The figure shows three views and two pictorial views of one solid part (mm, origin at its lowest corner). Answer the questions. A direction names the side the tool comes from. Coordinates: 2 decimals unless noted, no trailing zeros. Loops run counter-clockwise (first coordinate to the right, second up) from the corner with the lowest first, then second, coordinate; pieces in that order, holes last. Notation, with made-up numbers: (0.25, 33.5) - (38.25, 33.5) arc R17 ccw to (38.25, 63.5) - close; hole circle Ø7 at (34, -2). An arc over 180 degrees is marked (long way). One line per question, with ' | ' between items.
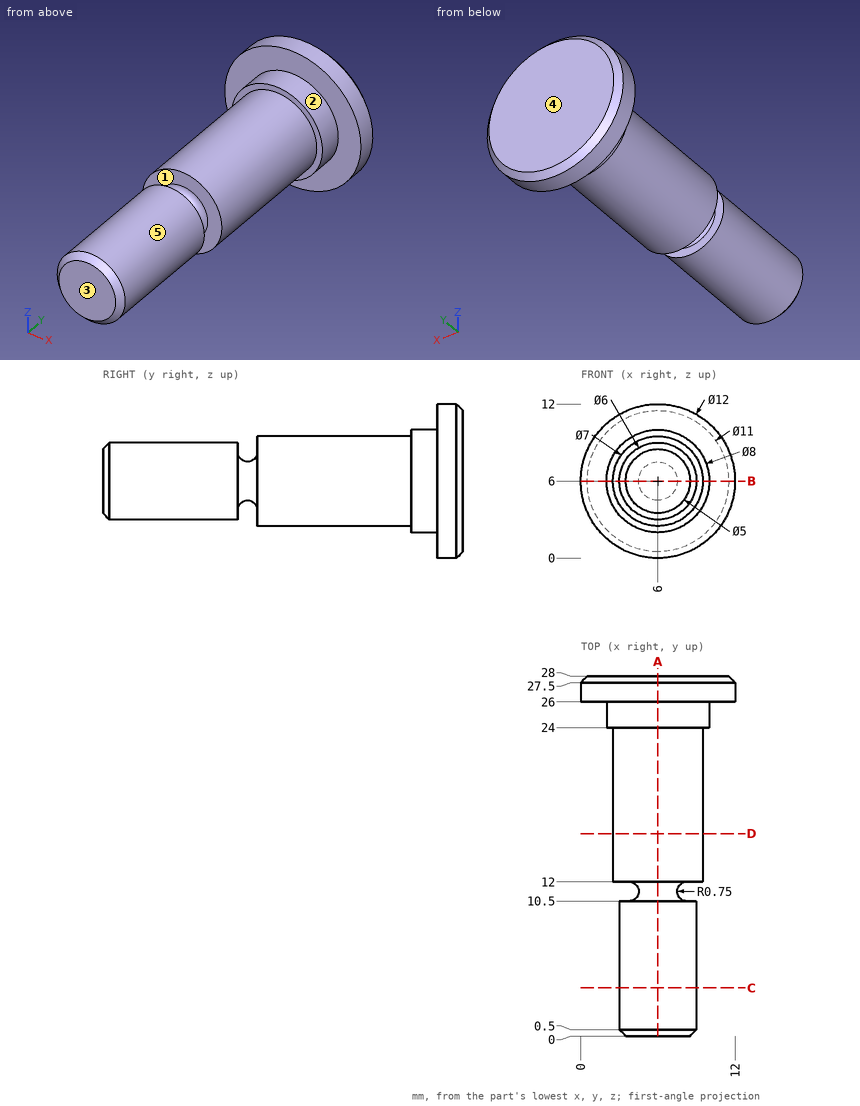
Item 1: Which of the six approach directions +Z, -Z, +X, -X, +Y, -Y give full straight-line access (tool end or side, diameter ignored) to the marked faces 4 and 5?
Taken from the geometry:
face 4: +Z, -Z, +X, -X, +Y | face 5: -Y
Item 2: Find section C-C, the plane y = 3.75. Write down the section's boundary in (x, z), plus the area to 3 significant figures.
Taken from the geometry:
outline: circle Ø6 at (6, 6) | area: 28.3 mm2
Item 3: Find section B-B, the plane z = 6. Write down the section's boundary in (x, y).
Taken from the geometry:
outline: (0, 26) - (2, 26) - (2, 24) - (2.5, 24) - (2.5, 12) - (3.75, 12) arc R0.75 cw to (3.75, 10.5) - (3, 10.5) - (3, 0.5) - (3.5, 0) - (8.5, 0) - (9, 0.5) - (9, 10.5) - (8.25, 10.5) arc R0.75 cw to (8.25, 12) - (9.5, 12) - (9.5, 24) - (10, 24) - (10, 26) - (12, 26) - (12, 27.5) - (11.5, 28) - (0.5, 28) - (0, 27.5) - close
Item 4: Find the intervals of material crossed by line 1 (Y direction, x = 2.5, z = 6.75); line 2 (Y direction, x = 10.5, z = 5.75); line 3 (X direction, y = 15, z = 6), in increasing order. Write a range as [from, to].
Taken from the geometry:
line 1: y = [24, 28] | line 2: y = [26, 28] | line 3: x = [2.5, 9.5]
Item 5: The mould has two halves that part along Y. Classify the marked faces 1, 2 and 3: pulls with the +Y half, pulls with the -Y half, needs draft (parallel to the pull), parting line crosses it, or undercut.
Taken from the geometry:
face 1: undercut | face 2: needs draft | face 3: pulls with the -Y half
Item 6: Each of these flat-tipped pins is pushed along its axis until it touches: pin 1 Ø6 at (x, z) = (6, 5.5) entering from -Y; pin 2 Ø1 at (x, y) = (7, 17.5) entering from +Z; pin 3 Ø1.5 at (y, z) = (22, 5.5) entering from -X; pin 4 Ø1 at (x, y) = (9, 10) entering from +Z. Where does it stop, or does it pass through?
Taken from the geometry:
pin 1: stops at y = 0 | pin 2: stops at z = 9.46 | pin 3: stops at x = 2.5 | pin 4: stops at z = 7.66
Item 7: Find section D-D, the plane y = 15.75. Write down the section's boundary in (x, z).
Taken from the geometry:
outline: circle Ø7 at (6, 6)
Item 8: Find section A-A, the plane x = 6. Write down the section's boundary in (y, z), plus the area to 3 significant figures.
Taken from the geometry:
outline: (0, 3.5) - (0.5, 3) - (10.5, 3) - (10.5, 3.75) arc R0.75 cw to (12, 3.75) - (12, 2.5) - (24, 2.5) - (24, 2) - (26, 2) - (26, 0) - (27.5, 0) - (28, 0.5) - (28, 11.5) - (27.5, 12) - (26, 12) - (26, 10) - (24, 10) - (24, 9.5) - (12, 9.5) - (12, 8.25) arc R0.75 cw to (10.5, 8.25) - (10.5, 9) - (0.5, 9) - (0, 8.5) - close | area: 191 mm2
